For this review, take the finished solid that the model builds, in its own axes (mm). A direction names the side the tool comes from. Give positions to 0.01 mm unless a question says otherwise; leave off trailing zeros. Order: outer loops, then holes, each group sorted by start corner. A loop starts at its lowest first (then second) coordinate and runs counter-clockwise, first axis right, second up. Notation, with made-up numbers: (59, -5) - (95, -5) arc R22 cw to (95, 10) - close; hole circle Ø10 at (81, 37). An arc over 180 degrees is marked (long way). One line per item, written item: value.
```python
from build123d import *

# Parameters (mm, degrees)
F1_DEPTH = 150
F2_W     = 51
F2_H     = 91
F2_W_2   = 45
F2_H_2   = 85
F3_DEPTH = 17
F4_DEPTH = 15
F5_W     = 85
F5_H     = 9
F6_DEPTH = 75
F7_W     = 45.0000017881
F7_H     = 9.0000017881
F8_DEPTH = 95


with BuildPart() as f1:
    # F0 (on Front) → F1 (new body)
    with BuildSketch(Plane.XZ):
        Polygon((-44.3471273035, 8.3293294263), (-29.3471273035, 8.3293294263), (-29.3471273035, 10.3293294263), (-30.6854649693, 10.3293294263), (-32.7072627842, 10.3293294263), (-44.3471273035, 10.3293294263), align=None)
        Polygon((-29.3471273035, -10.1195359603), (29.6528726965, -10.1195359603), (29.6528726965, 8.3293294263), (29.6528726965, 10.3293294263), (29.6528726965, 14.3293294263), (27.6528726965, 14.3293294263), (27.6528726965, 10.3293294263), (27.6528726965, 9.2171130797), (27.6528726965, -8.1195359603), (-27.3471273035, -8.1195359603), (-27.3471273035, 9.2171130797), (-27.3471273035, 10.3293294263), (-27.3471273035, 14.3293294263), (-29.3471273035, 14.3293294263), (-29.3471273035, 10.3293294263), (-29.3471273035, 8.3293294263), align=None)
        Polygon((29.6528726965, 10.3293294263), (29.6528726965, 8.3293294263), (44.6528726965, 8.3293294263), (44.6528726965, 10.3293294263), (41.5029401332, 10.3293294263), (33.3236008883, 10.3293294263), align=None)
    extrude(amount=-F1_DEPTH)

    # F2 (on face) → F3 (join)
    with BuildSketch(Plane.XY.offset(-8.1195359603)):
        with Locations((0, 75.1699954271)):
            Rectangle(F2_W, F2_H)
        with Locations((0, 75.1699954271)):
            Rectangle(F2_W_2, F2_H_2, mode=Mode.SUBTRACT)
        with Locations((0, 75.1699954271)):
            Rectangle(F2_W_2, F2_H_2)
    extrude(amount=-F3_DEPTH)

    # F2 (on face) → F4 (cut)
    with BuildSketch(Plane.XY.offset(-8.1195359603)):
        with Locations((0, 75.1699954271)):
            Rectangle(F2_W_2, F2_H_2)
    extrude(amount=-F4_DEPTH, mode=Mode.SUBTRACT)

    # F5 (on face) → F6 (cut)
    with BuildSketch(Plane.YZ.offset(25.5)):
        with Locations((75.1699954271, -17.6195359603)):
            Rectangle(F5_W, F5_H)
    extrude(amount=-F6_DEPTH, mode=Mode.SUBTRACT)

    # F7 (on face) → F8 (cut)
    with BuildSketch(Plane.XZ.offset(-29.6699954271)):
        with Locations((0, -17.6195359603)):
            Rectangle(F7_W, F7_H)
    extrude(amount=-F8_DEPTH, mode=Mode.SUBTRACT)


solid = f1.part
```
(1) For P1, Ø2, axis at y = 64, z = 12, coming from the -X side; P2, Ø10, axis at x = 20, z = -20.5, coming from the +Y side; P3, Ø18, axis at y = 85, z = -2, coming from the +X side; P4, Ø1.5, axis at x = 3, z = -20.5, coming from the -Y side, all flat-tipped, find the tip position at first contact; note any pin that passes through.
Answers below:
P1: stops at x = -29.35
P2: stops at y = 120.67
P3: stops at x = 29.65
P4: passes through
(2) Take a section at B-B (x = -18.5). Write out the cut boundary in (y, z), then the cut area to 3 significant figures.
Answers below:
outline: (0, -10.12) - (29.67, -10.12) - (29.67, -13.12) - (32.67, -13.12) - (32.67, -8.12) - (0, -8.12) - close; (29.67, -25.12) - (120.67, -25.12) - (120.67, -22.12) - (117.67, -22.12) - (117.67, -23.12) - (32.67, -23.12) - (32.67, -22.12) - (29.67, -22.12) - close; (117.67, -13.12) - (120.67, -13.12) - (120.67, -10.12) - (150, -10.12) - (150, -8.12) - (117.67, -8.12) - close
area: 336 mm^2
(3) Take a section at A-A (z = 2). Write out the cut boundary in (x, y).
Answers below:
outline: (-29.35, 0) - (-27.35, 0) - (-27.35, 150) - (-29.35, 150) - close; (27.65, 0) - (29.65, 0) - (29.65, 150) - (27.65, 150) - close
(4) Take a section at D-D (y = 15.5). Write out the cut boundary in (x, z).
Answers below:
outline: (-44.35, 8.33) - (-29.35, 8.33) - (-29.35, -10.12) - (29.65, -10.12) - (29.65, 8.33) - (44.65, 8.33) - (44.65, 10.33) - (29.65, 10.33) - (29.65, 14.33) - (27.65, 14.33) - (27.65, -8.12) - (-27.35, -8.12) - (-27.35, 14.33) - (-29.35, 14.33) - (-29.35, 10.33) - (-44.35, 10.33) - close
(5) Wall thickness on line 1 (X direction, y = 56, z = -6); line 2 (Z direction, x = 12, y = 118); line 3 (X direction, y = 31, z = -16): over which ranges is each line inside the solid? List them lowest first. Write a range as from..to.
Answers below:
line 1: x = -29.35..-27.35, 27.65..29.65
line 2: z = -25.12..-22.12, -13.12..-8.12
line 3: x = -25.5..-22.5, 22.5..25.5
(6) Draft analysis for pull direction X (two halves, no side actions). For faces 1 (the face through (0, 120.67, -23)), 2 (the face through (22.5, 31, -18)), 3 (the face through (25.5, 75, -23)), 4 (the face through (0, 117.67, -11)), state which applies: pulls with the +X half, pulls with the -X half, needs draft (parallel to the pull), parting line crosses it, or undercut.
Answers below:
face 1: needs draft
face 2: undercut
face 3: pulls with the +X half
face 4: undercut
(7) Machinability: for faces 5 (the face through (-29.347, 74, -1)), 6 (the face through (24, 75, -22.12)), 7 (the face through (-22.5, 31, -18)), which of the approach directions +Z, -Z, +X, -X, +Y, -Y give a long, thin tool a straight path to every point of the face, cutting with its end or side? Answer none if there is none.
Answers below:
face 5: -Z, -X, +Y, -Y
face 6: +X, -X
face 7: +Y, -Y
(8) Take a section at C-C (z = -15). Write out the cut boundary in (x, y).
Answers below:
outline: (-25.5, 29.67) - (-22.5, 29.67) - (-22.5, 32.67) - (-25.5, 32.67) - close; (-25.5, 117.67) - (-22.5, 117.67) - (-22.5, 120.67) - (-25.5, 120.67) - close; (22.5, 29.67) - (25.5, 29.67) - (25.5, 32.67) - (22.5, 32.67) - close; (22.5, 117.67) - (25.5, 117.67) - (25.5, 120.67) - (22.5, 120.67) - close
